Study the drawing (mm; zero at the part's minimum x, y, z) and answer. Round coordinates to 2 decimals unless told otherwise and drop trailing zeros. Loops run counter-clockwise (first coordinate to the right, second up) from the corner with the lowest first, then second, coordinate; pieces in that order, holes last. Notation, with made-up numbers: (62, 56) -> (83, 56) arc R26 ccw to (83, 89) -> close; hole circle Ø7 at (-0.75, 17.25). An arc over 180 degrees is marked (long way). Write each question's results on one line, items separated by ' | '. Start each with the question number.
(1) The part is cut by section B-B (x = 9). Determine the outline of the cut face in (y, z) (1 decimal), plus the area to 3 significant figures.
(2) The part is cut by section A-A (z = 14). Determine the outline of the cut face in (x, y) (1 decimal).
(3) The part is cut by section C-C (y = 0.7). Count the separate pieces of the cut face and the enclosed holes in it, plus the area to 3 significant figures.
(4) A flat-ended cylindrical pin translates along its axis: pin 1 (0.9 mm diameter, centred on x = 1.55, z = 1.14, fed in from +Y). Find the tip coordinate at first contact, or state that the pin passes through.
(5) Straight lines are drawn through the part: probe 1 along X at (y, z) = (0.95, 13.25) (1 decimal); probe 2 along X at (y, z) = (0.9, 14.5) (1 decimal); probe 3 along Z at (x, y) = (3.25, 0.6) (1 decimal). For each, find the intervals that lie inside material, in ascending order.
(6) The part is cut by section D-D (x = 18). Determine the outline of the cut face in (y, z).
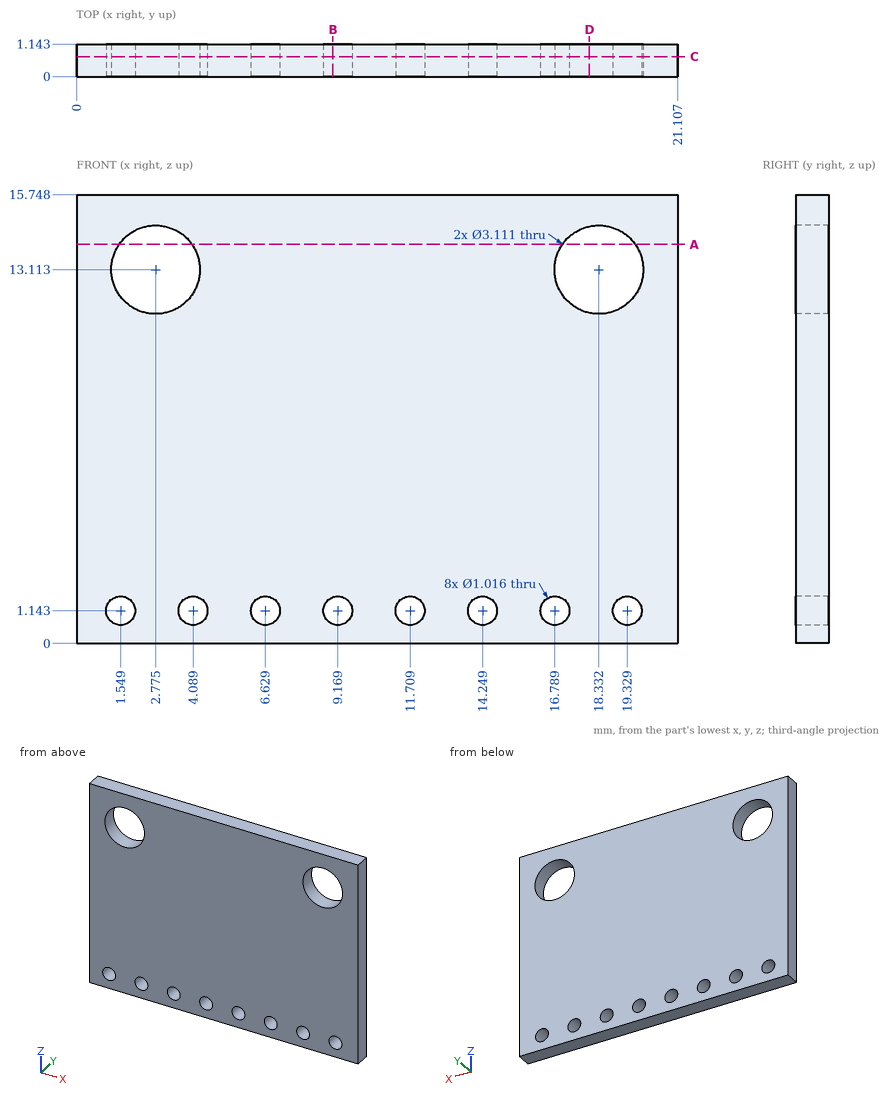
Checked values:
1) outline: (0, 0) -> (1.1, 0) -> (1.1, 0.7) -> (0, 0.7) -> close; (0, 1.6) -> (1.1, 1.6) -> (1.1, 15.7) -> (0, 15.7) -> close | area: 16.9 mm2
2) outline: (0, 0) -> (1.5, 0) -> (1.5, 1.1) -> (0, 1.1) -> close; (4.1, 0) -> (17.1, 0) -> (17.1, 1.1) -> (4.1, 1.1) -> close; (19.6, 0) -> (21.1, 0) -> (21.1, 1.1) -> (19.6, 1.1) -> close
3) separate pieces: 1 | enclosed holes: 10 | area: 311 mm2
4) pin 1: passes through
5) probe 1: x = 0 to 1.2, 4.3 to 16.8, 19.9 to 21.1 | probe 2: x = 0 to 2.1, 3.5 to 17.6, 19 to 21.1 | probe 3: z = 0 to 11.6, 14.6 to 15.7
6) outline: (0, 0) -> (1.14, 0) -> (1.14, 11.59) -> (0, 11.59) -> close; (0, 14.63) -> (1.14, 14.63) -> (1.14, 15.75) -> (0, 15.75) -> close
